```python
from build123d import *

# Parameters (mm, degrees)
F0_W     = 69.685258
F0_H     = 69.96853
F1_DEPTH = 100
F2_W     = 69.685258
F2_H     = 61.617006
F3_DEPTH = 90
F4_W     = 63.10162
F4_H     = 22.249703
F5_DEPTH = 25


with BuildPart() as f1:
    # F0 (on Front) → F1 (new body)
    with BuildSketch(Plane.XZ):
        Rectangle(F0_W, F0_H)
    extrude(amount=F1_DEPTH)

    # F2 (on face) → F3 (cut)
    with BuildSketch(Plane(origin=(0, 0, 0), x_dir=(-1, 0, 0), z_dir=(0, 1, 0))):
        with Locations((0, 4.175762)):
            Rectangle(F2_W, F2_H)
    extrude(amount=-F3_DEPTH, mode=Mode.SUBTRACT)

    # F4 (on face) → F5 (cut)
    with BuildSketch(Plane.XZ.offset(100)):
        with Locations((0.287328, 20.602283)):
            Rectangle(F4_W, F4_H)
    extrude(amount=-F5_DEPTH, mode=Mode.SUBTRACT)


solid = f1.part
```
Geometry check sheet. Reference: the model listing, model coordinates, mm. A direction names the side the tool comes from. Coordinates: 2 decimals unless noted, no trailing zeros. Loops run counter-clockwise (first coordinate to the right, second up) from the corner with the lowest first, then second, coordinate; pieces in that order, holes last.
Item 1: Sectioned sample at C-C, the plane y = -66. Record the boundary of the cut face in (x, z), then the cut area to 3 significant figures.
Item 2: Access from +Z, -Z, +X, -X, +Y, -Y to the whole of each face (thin tool, end or side, straight path). Record for faces 1 (the face through (0, -95, 31.727)), 2 (the face through (0, -44, -26.633)), 3 (the face through (0, -49, -34.984)).
Item 3: Sectioned sample at B-B, the plane z = 25. Record the boundary of the cut face in (x, y).
Item 4: Sectioned sample at D-D, the plane z = -4. Record the boundary of the cut face in (x, y).
Item 5: Thickness scan on line 1 (Z direction, x = -25, y = -95); line 2 (Z direction, x = 2.5, y = -46.5); line 3 (Y direction, x = -4.5, z = -0.5). Record the ranges inside material, lowest first.
Item 6: Sectioned sample at A-A, the plane x = 8.5. Record the boundary of the cut face in (y, z), then the cut area to 3 significant figures.
Item 7: Release check for a two-part mould opening along X. For faces 4 (the face through (34.843, -72, -29)), 5 (the face through (0, -95, 34.984)), 6 (the face through (0, -95, 9.477)) record: released by +X, released by -X, zero draft, split by the parting line, or undercut.
Item 8: Go/stop test with flat-tipped pins: pin 1 Ø5 at (x, y) = (19.5, -22) entering from +Z; pin 2 Ø8 at (x, z) = (0.5, -13.5) entering from +Y. Record where each tip stops, or that it passes through.
Check result:
1. outline: (-34.84, -34.98) - (34.84, -34.98) - (34.84, -26.63) - (-34.84, -26.63) - close
1. area: 582 mm2
2. face 1: +Y, -Y
2. face 2: +Z, +X, -X, +Y
2. face 3: -Z, +X, -X, +Y, -Y
3. outline: (-34.84, -100) - (-31.26, -100) - (-31.26, -90) - (-34.84, -90) - close; (31.84, -100) - (34.84, -100) - (34.84, -90) - (31.84, -90) - close
4. outline: (-34.84, -100) - (34.84, -100) - (34.84, -90) - (-34.84, -90) - close
5. line 1: z = -34.98 to 9.48, 31.73 to 34.98
5. line 2: z = -34.98 to -26.63
5. line 3: y = -100 to -90
6. outline: (-100, -34.98) - (0, -34.98) - (0, -26.63) - (-90, -26.63) - (-90, 9.48) - (-100, 9.48) - close; (-100, 31.73) - (-90, 31.73) - (-90, 34.98) - (-100, 34.98) - close
6. area: 1,230 mm2
7. face 4: released by +X
7. face 5: zero draft
7. face 6: undercut
8. pin 1: stops at z = -26.63
8. pin 2: stops at y = -90
